Check sheet for the drawn part. Datum: minimum x, y, z corner. Units: mm. A direction names the side the tool comes from. Round coordinates to 2 decimals unless told otherwise and drop trailing zeros. Order: outer loops, then holes, each group sorted by start corner. A loop starts at its lowest first (then second) coordinate and runs counter-clockwise, first axis right, second up. Notation, with made-up numbers: (84.5, 4) -> (140.5, 4) arc R21 ccw to (140.5, 16) -> close; hole circle Ø10 at (26.25, -19.75). An arc over 180 degrees is marked (long way). Answer as CSV lines item,"result". Start each with the question number.
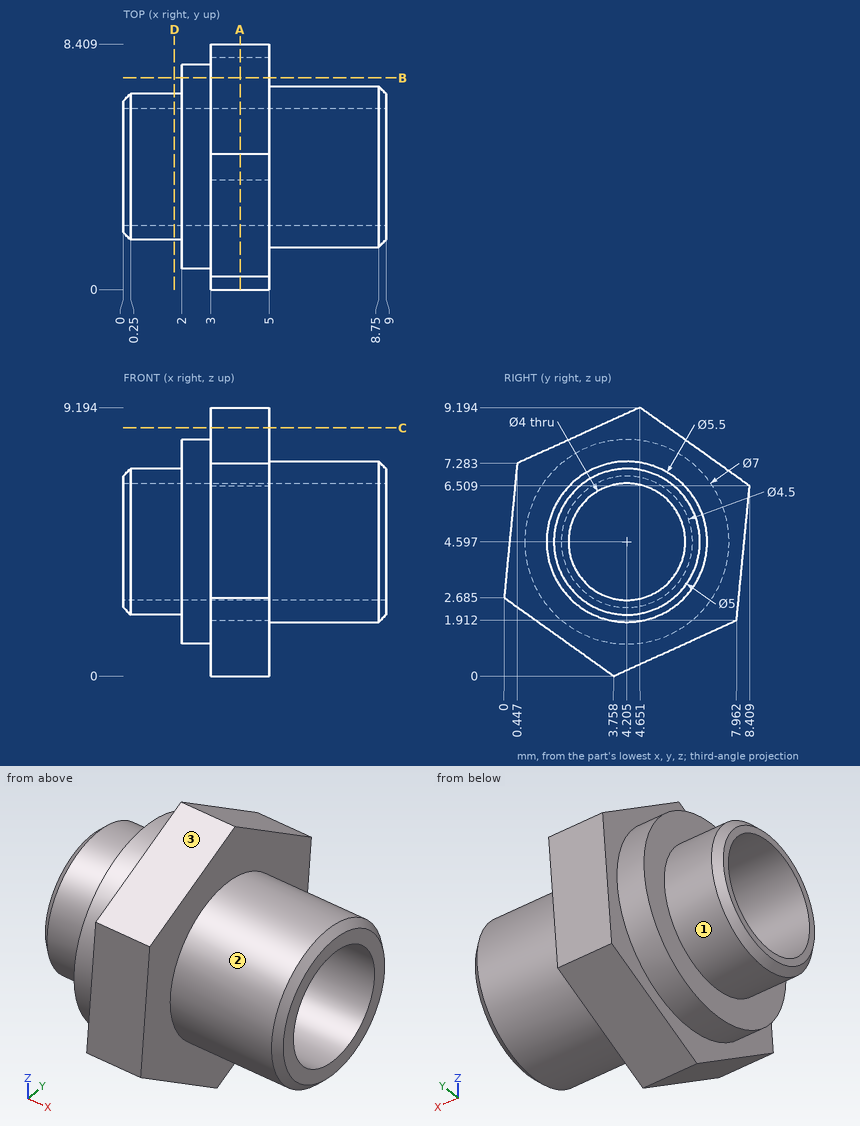
1) Section check C-C on z = 8.5. Record the cut outline in (x, y) (1 decimal).
2) Section check B-B on y = 7.25. Record the cut outline in (x, z).
3) Depth check by flat-ended pin: pin 1 Ø2 at (y, z) = (4.5, 1.5) entering from -X; pin 2 Ø1.5 at (x, y) = (3.5, 1.5) entering from +Z. Enter the tip coordinate at first touch or a pass-through.
4) Section check A-A on x = 4. Record the cut outline in (y, z) (1 decimal).
5) Material ranges on line 1 along X through (y, z) = (7.5, 3.25); line 2 along X through (y, z) = (7, 5.75); line 3 along Y through (x, z) = (3.5, 1.25) (1 decimal), recorded low to high.
6) Section check D-D on x = 1.75. Record the cut outline in (y, z) (1 decimal).
7) Access from +Z, -Z, +X, -X, +Y, -Y to the whole of each face (thin tool, end or side, straight path). Record for the marked faces 1, 2 and 3.
Solutions:
1,outline,"(3, 3.1) -> (5, 3.1) -> (5, 5.6) -> (3, 5.6) -> close"
2,outline,"(2, 2.87) -> (3, 2.87) -> (3, 1.59) -> (5, 1.59) -> (5, 7.34) -> (3, 7.34) -> (3, 6.32) -> (2, 6.32) -> close"
3,pin 1,"stops at x = 0"
3,pin 2,"stops at z = 8.1"
4,outline,"(0, 2.7) -> (3.8, 0) -> (8, 1.9) -> (8.4, 6.5) -> (4.7, 9.2) -> (0.4, 7.3) -> close; hole circle Ø4 at (4.2, 4.6)"
5,line 1,"x = 3 to 5"
5,line 2,"x = 2 to 5"
5,line 3,"y = 2 to 6.5"
6,outline,"circle Ø5 at (4.2, 4.6); hole circle Ø4 at (4.2, 4.6)"
7,face 1,"-X"
7,face 2,"+X"
7,face 3,"+Z, +X, -X, -Y"
